Answer from the drawing. Dimensions are ordinates in mm from the lowest x, y and z of the part. A direction names the side the tool comes from. Round coordinates to 2 decimals unless told otherwise and drop trailing zeros. Loops run counter-clockwise (first coordinate to the right, second up) from the corner with the lowest first, then second, coordinate; pieces in that order, holes last. Notation, with made-up numbers: (84, -6) - (141, -6) arc R23 ccw to (141, 19) - close; hole circle Ø7 at (1, -4). An arc over 180 degrees is marked (long way). Write item = value, one per line. Start each with the question number.
1) A tool of negligible diameter and unlimited length cuts with its end or side. For the marked faces 4 and 5, from which of +Z, -Z, +X, -X, +Y, -Y can it reach the whole face along a straight path? Write none if from no direction.
2) Section C-C, the plane z = 24 is taken. Determine the outline of the cut face in (x, y), and give its area (3 significant figures).
3) Straight lines are drawn through the part: line 1 along X through (y, z) = (98.4, 10); line 2 along Y through (x, z) = (24, 14). For each, find the intervals that lie inside material, in ascending order.
4) For a pull along X with two mould halves and no side action, classify the marked faces 1, 2 and 3 as released by +X, released by -X, zero draft, split by the parting line, or undercut.
5) Section B-B, the plane x = 34 is taken. Determine the outline of the cut face in (y, z).
6) Given pin 1 Ø1.6 at (x, z) = (15, 10) entering from -Y; pin 2 Ø11.5 at (x, y) = (50, 50) entering from +Z, each flat-ended and moving along its own axis, determine where each tip first touches the part or whether it passes through.
7) Section A-A, the plane y = 50 is taken. Determine the outline of the cut face in (x, z), and give its area (3 significant figures).
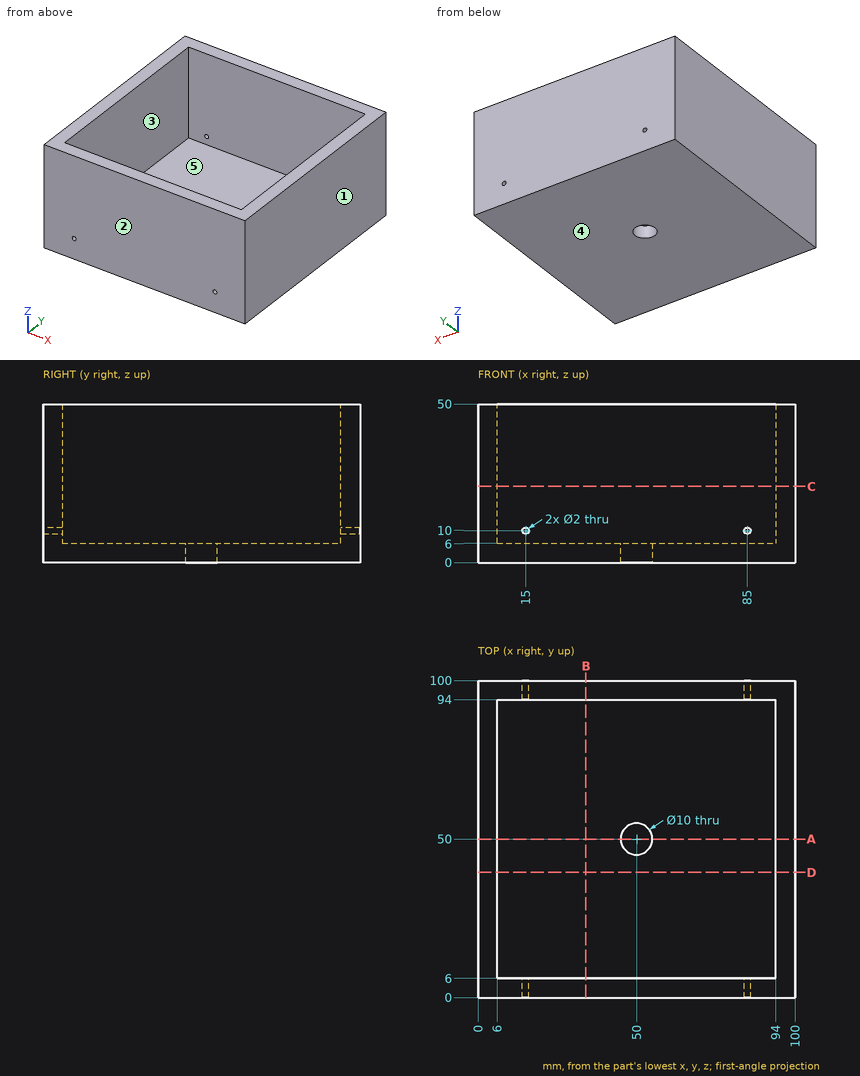
Geometry check:
q1.face_4 = -Z, +X, -X, +Y, -Y
q1.face_5 = +Z
q2.outline = (0, 0) - (100, 0) - (100, 100) - (0, 100) - close; hole (6, 6) - (94, 6) - (94, 94) - (6, 94) - close
q2.area = 2,260 mm2
q3.line_1 = 0 to 14, 16 to 84, 86 to 100
q3.line_2 = 0 to 6, 94 to 100
q4.face_1 = released by +X
q4.face_2 = zero draft
q4.face_3 = undercut
q5.outline = (0, 0) - (100, 0) - (100, 50) - (94, 50) - (94, 6) - (6, 6) - (6, 50) - (0, 50) - close
q6.pin_1 = through
q6.pin_2 = 6
q7.outline = (0, 0) - (45, 0) - (45, 6) - (6, 6) - (6, 50) - (0, 50) - close; (55, 0) - (100, 0) - (100, 50) - (94, 50) - (94, 6) - (55, 6) - close
q7.area = 1,070 mm2
